Autodesk Inventor part; units mm, degrees
ref_plane "YZ Plane" through (0, 0, 0) normal (1, 0, 0) x (0, 1, 0)
ref_plane "XY Plane" through (0, 0, 0) normal (0, 0, 1) x (1, 0, 0)
sketch "Sketch1" plane through (0, 0, 0) normal (0, 0, 1) x (1, 0, 0)
  line L0 (-150, -150) -> (150, -150)
  line L1 (150, -150) -> (150, 150)
  line L2 (150, 150) -> (-150, 150)
  line L3 (-150, 150) -> (-150, -150)
  line L4 (-150, -150) -> (150, 150) construction
  line L5 (150, -150) -> (-150, 150) construction
  point P0 (0, 0)
  dimension "d0" = 300
  dimension "d1" = 300
extrude "Extrusion1" add sketch "Sketch1" along normal blind 50
sketch "Sketch2" plane through (0, 0, 50) normal (0, 0, 1) x (1, 0, 0)
  circle A0 centre (0, 0) radius 100
  dimension "D_agujero" = 200
extrude "Extrusion2" cut sketch "Sketch2" against normal through all
ref_plane "Work Plane1" through (0, 100, 50) normal (0, 1, 0) x (-1, 0, 0)
equation "\"d0\" = 1.5 * tamanio_basico"
equation "\"d1\" = 1.5 * tamanio_basico"
equation "\"espesor\" = 0.25 * tamanio_basico"
equation "\"D_agujero\" = tamanio_basico"
equation "\"tamanio_basico\" = 200"
properties part number "AGUJERO"
Geometry check sheet. Reference: the model listing, model coordinates, mm. Round coordinates to 2 decimals unless told otherwise and drop trailing zeros. Order: outer loops, then holes, each group sorted by start corner. A loop starts at its lowest first (then second) coordinate and runs counter-clockwise, first axis right, second up. Notation, with made-up numbers: (55.25, 27) - (111.25, 27) arc R20 cw to (111.25, 66) - close; hole circle Ø3 at (8, 80). An arc over 180 degrees is marked (long way). Use a Markdown table: item, result. Add a question column.
1) Gauge pin test, flat end, axial feed: P1, Ø1.5, axis at x = 78, y = -98.5, coming from the -Z side. Record the tip position at first contact, or that the pin passes through.
2) Thickness scan on line 1 along Y through (x, z) = (0, 13); line 2 along X through (y, z) = (90.5, 42.5); line 3 along Y through (x, z) = (62, 44.5). Record the ranges inside material, lowest first.
3) Mould release check, pull along X, two halves, no side actions. Record for faces 1 (the flat face through (-2, 102, 0)), 2 (the flat face through (150, -2, 25)), 3 (the cylindrical face through (95.38, 30.04, 25.35)): released by +X, released by -X, zero draft, split by the parting line, or undercut.
4) Section check C-C (z = 41). Record the cut outline in (x, y).
5) Section check A-A (y = 0). Record the cut outline in (x, z).
Established:
| question | item | result |
|---|---|---|
| 1 | P1 | z = 0 |
| 2 | line 1 | -150 to -100, 100 to 150 |
| 2 | line 2 | -150 to -42.54, 42.54 to 150 |
| 2 | line 3 | -150 to -78.46, 78.46 to 150 |
| 3 | face 1 | zero draft |
| 3 | face 2 | released by +X |
| 3 | face 3 | undercut |
| 4 | outline | (-150, -150) - (150, -150) - (150, 150) - (-150, 150) - close; hole circle Ø200 at (0, 0) |
| 5 | outline | (-150, 0) - (-100, 0) - (-100, 50) - (-150, 50) - close; (100, 0) - (150, 0) - (150, 50) - (100, 50) - close |
